The listing builds one solid part. Answer for the finished solid, in the listing's coordinates (mm). Face numbers are marked on the shaded views. A direction names the side the tool comes from. Coordinates: 2 decimals unless noted, no trailing zeros. Order: outer loops, then holes, each group sorted by start corner. A loop starts at its lowest first (then second) coordinate and runs counter-clockwise, first axis right, second up. Notation, with made-up numbers: (28.5, -29.75) -> (37.5, -29.75) arc R11 ccw to (37.5, -16.75) -> close; hole circle Ø4 at (12.5, 49). An arc over 180 degrees is marked (long way). Put each result on its own line as item: value. Start each with the question number.
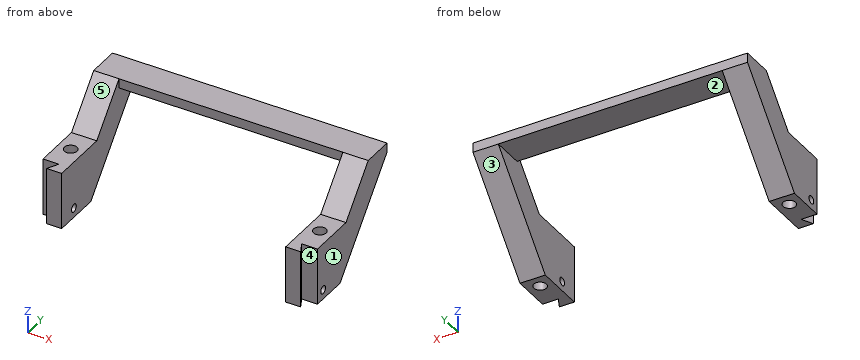
```python
from build123d import *

# Parameters (mm, degrees)
BOSS_EXTRUDE1_DEPTH   = 8
CUT_EXTRUDE2_DEPTH    = 53.318734694
M3X0_5_TAPPED_HOLE1_D = 2.5
SKETCH7_W             = 3
SKETCH7_H             = 10
BOSS_EXTRUDE2_DEPTH   = 4
SKETCH8_W             = 3
SKETCH8_H             = 10
BOSS_EXTRUDE3_DEPTH   = 66.83
SKETCH10_R            = 2
CUT_EXTRUDE3_DEPTH    = 91.659632141
SKETCH11_R            = 2
CUT_EXTRUDE4_DEPTH    = 91.659632141
SKETCH12_W            = 8
SKETCH12_H            = 0.5
CUT_EXTRUDE5_DEPTH    = 95.273108043
SKETCH13_W            = 8
SKETCH13_H            = 0.5
CUT_EXTRUDE6_DEPTH    = 95.273108043


with BuildPart() as part:
    # Sketch1 → Boss-Extrude1 (new body)
    with BuildSketch(Plane(origin=(0, 0, 0), x_dir=(0, 0, -1), z_dir=(1, 0, 0))):
        Polygon((0, 0), (0, 16), (-28.5, 41), (-31.5, 41), (-31.5, 31), (-18, 19.157894737), (-18, 0), align=None)
    boss_extrude1 = extrude(amount=BOSS_EXTRUDE1_DEPTH)

    # Sketch3 → Cut-Extrude2 (cut, through all)
    with BuildSketch(Plane(origin=(0, 0, 0), x_dir=(-1, 0, 0), z_dir=(0, 0, -1))):
        Polygon((-8, 0), (-5, 0), (-3, 4), (-8, 4), align=None)
    cut_extrude2 = extrude(amount=-CUT_EXTRUDE2_DEPTH, mode=Mode.SUBTRACT)

    # M3x0.5 Tapped Hole1 (through all)
    with Locations(Plane(origin=(8, 7, 3), x_dir=(0, 0, 1), z_dir=(1, 0, 0))):
        with Locations((0, 0)):
            m3x0_5_tapped_hole1 = Hole(M3X0_5_TAPPED_HOLE1_D / 2)

    # Sketch7 → Boss-Extrude2 (add)
    with BuildSketch(Plane.ZY):
        with Locations((30, 36)):
            Rectangle(SKETCH7_W, SKETCH7_H)
    extrude(amount=BOSS_EXTRUDE2_DEPTH)

    # Sketch8 → Boss-Extrude3 (add)
    with BuildSketch(Plane.ZY.offset(4)):
        with Locations((30, 36)):
            Rectangle(SKETCH8_W, SKETCH8_H)
    extrude(amount=BOSS_EXTRUDE3_DEPTH)

    # Mirror1: Boss-Extrude1, Cut-Extrude2, M3x0.5 Tapped Hole1 across plane
    add(boss_extrude1.mirror(Plane.ZY.offset(35.415)))
    add(cut_extrude2.mirror(Plane.ZY.offset(35.415)), mode=Mode.SUBTRACT)
    add(m3x0_5_tapped_hole1.mirror(Plane.ZY.offset(35.415)), mode=Mode.SUBTRACT)

    # Sketch10 → Cut-Extrude3 (cut, through all)
    with BuildSketch(Plane.XY.offset(18)):
        with Locations((4, 12)):
            Circle(SKETCH10_R)
    extrude(amount=-CUT_EXTRUDE3_DEPTH, mode=Mode.SUBTRACT)

    # Sketch11 → Cut-Extrude4 (cut, through all)
    with BuildSketch(Plane.XY.offset(18)):
        with Locations((-74.83, 12)):
            Circle(SKETCH11_R)
    extrude(amount=-CUT_EXTRUDE4_DEPTH, mode=Mode.SUBTRACT)

    # Sketch12 → Cut-Extrude5 (cut, through all)
    with BuildSketch(Plane(origin=(0, 0, 0), x_dir=(-1, 0, 0), z_dir=(0, 0, -1))):
        with Locations((-4, 0.25)):
            Rectangle(SKETCH12_W, SKETCH12_H)
    extrude(amount=-CUT_EXTRUDE5_DEPTH, mode=Mode.SUBTRACT)

    # Sketch13 → Cut-Extrude6 (cut, through all)
    with BuildSketch(Plane(origin=(0, 0, 0), x_dir=(-1, 0, 0), z_dir=(0, 0, -1))):
        with Locations((74.83, 0.25)):
            Rectangle(SKETCH13_W, SKETCH13_H)
    extrude(amount=-CUT_EXTRUDE6_DEPTH, mode=Mode.SUBTRACT)


solid = part.part
```
(1) Find the intervals of material crossed by L1, parallel to X at y = 7.5, z = 9; L2, parallel to Y at x = 4, z = 6; L3, parallel to Z at x = -63, y = 34, in increasing order.
(2) A tool of negligible diameter and unlimited length cuts with its end or side. For the marked faces 4 and 5, from which of +Z, -Z, +X, -X, +Y, -Y can it reach the whole face along a straight path? Write none if from no direction.
(3) The part is cut by section B-B on z = 14.5. Determine the outline of the cut face in (x, y).
(4) The part is cut by section A-A on y = 12. Determine the outline of the cut face in (x, z).
(5) The part is cut by section C-C on y = 25. Determine the outline of the cut face in (x, z).
(6) For a pull along X with two mould halves and no side action, classify the marked faces 1, 2 and 3 as released by +X, released by -X, zero draft, split by the parting line, or undercut.
(7) The part is cut by section D-D on z = 3. Determine the outline of the cut face in (x, y).
(8) Each of these flat-tipped pins is pushed along its axis until it touches: P1, Ø5, axis at x = -38, y = 35, coming from the -Z side; P2, Ø4, axis at x = -76, y = 5, coming from the +Z side; P3, Ø3.5, axis at x = -50, z = 30.5, coming from the -Y side. Where does it stop, or does it pass through?
Worked out:
1. L1: -78.83 to -70.83, 0 to 8
1. L2: 0.5 to 2, 4 to 10, 14 to 21.26
1. L3: 28.5 to 31.5
2. face 4: +Z, -Z, +X
2. face 5: +Z, +X, -X, -Y
3. outline: (-78.83, 4) -> (-73.83, 4) -> (-75.58, 0.5) -> (-70.83, 0.5) -> (-70.83, 28.72) -> (-78.83, 28.72) -> close; (0, 0.5) -> (4.75, 0.5) -> (3, 4) -> (8, 4) -> (8, 28.72) -> (0, 28.72) -> close; hole circle Ø4 at (-74.83, 12); hole circle Ø4 at (4, 12)
4. outline: (-78.83, 0) -> (-76.83, 0) -> (-76.83, 18) -> (-78.83, 18) -> close; (-72.83, 0) -> (-70.83, 0) -> (-70.83, 18) -> (-72.83, 18) -> close; (0, 0) -> (2, 0) -> (2, 18) -> (0, 18) -> close; (6, 0) -> (8, 0) -> (8, 18) -> (6, 18) -> close
5. outline: (-78.83, 10.26) -> (-70.83, 10.26) -> (-70.83, 24.66) -> (-78.83, 24.66) -> close; (0, 10.26) -> (8, 10.26) -> (8, 24.66) -> (0, 24.66) -> close
6. face 1: released by +X
6. face 2: undercut
6. face 3: zero draft
7. outline: (-78.83, 4) -> (-73.83, 4) -> (-75.58, 0.5) -> (-70.83, 0.5) -> (-70.83, 5.75) -> (-78.83, 5.75) -> close; (-78.83, 8.25) -> (-70.83, 8.25) -> (-70.83, 18.63) -> (-78.83, 18.63) -> close; (0, 0.5) -> (4.75, 0.5) -> (3, 4) -> (8, 4) -> (8, 5.75) -> (0, 5.75) -> close; (0, 8.25) -> (8, 8.25) -> (8, 18.63) -> (0, 18.63) -> close; hole circle Ø4 at (-74.83, 12); hole circle Ø4 at (4, 12)
8. P1: z = 28.5
8. P2: z = 18
8. P3: y = 31
